Can you work these out from the model? Positions are in its coordinate system, mm. A direction names the side the tool comes from. Give positions to 0.01 mm unless a question says otherwise; leave off trailing zeros. Write each loop counter-clockwise with the first axis right and the second up, starting at its lowest first coordinate (ties: lowest second). Pieces come first, ordered by that corner, then holes.
from build123d import *

# Parameters (mm, degrees)
SKETCH1_W           = 50
SKETCH1_H           = 25
BOSS_EXTRUDE2_DEPTH = 3
SKETCH3_R           = 8.25
CUT_EXTRUDE2_DEPTH  = 29.111385594
SKETCH6_W           = 50
SKETCH6_H           = 25
SKETCH6_W_2         = 46
SKETCH6_H_2         = 21
BOSS_EXTRUDE3_DEPTH = 6
SKETCH7_W           = 50
SKETCH7_H           = 2
BOSS_EXTRUDE4_DEPTH = 12
SKETCH9_R           = 1.5
CUT_EXTRUDE3_DEPTH  = 40.937451095


with BuildPart() as part:
    # Sketch1 → Boss-Extrude2 (new body)
    with BuildSketch(Plane(origin=(0, 0, 0), x_dir=(1, 0, 0), z_dir=(0, 1, 0))):
        Rectangle(SKETCH1_W, SKETCH1_H)
    extrude(amount=BOSS_EXTRUDE2_DEPTH)

    # Sketch3 → Cut-Extrude2 (cut, through all)
    with BuildSketch(Plane(origin=(0, 3, 0), x_dir=(1, 0, 0), z_dir=(0, 1, 0))):
        with Locations(Location((13.25, 0, 0), (0, 0, 270))):
            Circle(SKETCH3_R)
        with Locations(Location((-13.25, 0, 0), (0, 0, 270))):
            Circle(SKETCH3_R)
    extrude(amount=-CUT_EXTRUDE2_DEPTH, mode=Mode.SUBTRACT)

    # Sketch6 → Boss-Extrude3 (add)
    with BuildSketch(Plane(origin=(0, 3, 0), x_dir=(1, 0, 0), z_dir=(0, 1, 0))):
        Rectangle(SKETCH6_W, SKETCH6_H)
        Rectangle(SKETCH6_W_2, SKETCH6_H_2, mode=Mode.SUBTRACT)
    extrude(amount=BOSS_EXTRUDE3_DEPTH)

    # Sketch7 → Boss-Extrude4 (add)
    with BuildSketch(Plane(origin=(0, 9, 0), x_dir=(1, 0, 0), z_dir=(0, 1, 0))):
        with Locations((0, -11.5)):
            Rectangle(SKETCH7_W, SKETCH7_H)
    extrude(amount=BOSS_EXTRUDE4_DEPTH)

    # Sketch9 → Cut-Extrude3 (cut, through all)
    with BuildSketch(Plane(origin=(0, 0, 10.5), x_dir=(-1, 0, 0), z_dir=(0, 0, -1))):
        with Locations((-15, 15.02673795)):
            Circle(SKETCH9_R)
        with Locations((15, 15.02673795)):
            Circle(SKETCH9_R)
    extrude(amount=-CUT_EXTRUDE3_DEPTH, mode=Mode.SUBTRACT)


solid = part.part
(1) Imagine slicing it at A-A, the plane z = 0. Write out the boundary of the cut face in (x, y), plus the area to 3 significant figures.
Returned:
outline: (-25, 0) - (-21.5, 0) - (-21.5, 3) - (-23, 3) - (-23, 9) - (-25, 9) - close; (-5, 0) - (5, 0) - (5, 3) - (-5, 3) - close; (21.5, 0) - (25, 0) - (25, 9) - (23, 9) - (23, 3) - (21.5, 3) - close
area: 75.0 mm2
(2) Will these pins go through, and if not, where does the flat tip stop? P1, Ø1.8, axis at x = 15, y = 15.03, coming from the +Z side; P2, Ø7, axis at x = -1, z = 2, coming from the +Y side.
Returned:
P1: passes through
P2: stops at y = 3
(3) Imagine slicing it at D-D, the plane x = 22.5. Write out the boundary of the cut face in (y, z), plus the area to 3 significant figures.
Returned:
outline: (0, -12.5) - (9, -12.5) - (9, -10.5) - (3, -10.5) - (3, 10.5) - (21, 10.5) - (21, 12.5) - (0, 12.5) - close
area: 123 mm2
(4) For faces 5 (the face through (5.2, 1.5, -1.8)), 6 (the face through (-2, 9, -11)), 7 (the face through (0, 3, 0)), which set-ups out of +Z, -Z, +X, -X, +Y, -Y let a thin tool reach every point of the face, with its end or its side?
Returned:
face 5: +Y, -Y
face 6: -Z, +X, -X, +Y
face 7: +Y
(5) If we mould it in two halves opening along X, with no side actions, what happens to faces 1 (the face through (23, 6, 0)), 2 (the face through (0, 6, -10.5)), 3 (the face through (0, 0, 0)), 4 (the face through (25, 6, 0))? For each: +X half, -X half, draft (parallel to the pull), parting line (faces both ways), or undercut.
Returned:
face 1: undercut
face 2: undercut
face 3: draft
face 4: +X half
(6) If I drill on L1, parallel to X at y = 1.5, z = 0; L2, parallel to Y at x = 15, z = 11.7; L3, parallel to X at y = 2.25, z = -4, over which ranges is the centre line in solid material (lowest first)?
Returned:
L1: x = -25 to -21.5, -5 to 5, 21.5 to 25
L2: y = 0 to 13.53, 16.53 to 21
L3: x = -25 to -20.47, -6.03 to 6.03, 20.47 to 25
(7) Imagine slicing it at C-C, the plane y = 7.5. Write out the boundary of the cut face in (x, z), plus the area to 3 significant figures.
Returned:
outline: (-25, -12.5) - (25, -12.5) - (25, 12.5) - (-25, 12.5) - close; hole (-23, -10.5) - (23, -10.5) - (23, 10.5) - (-23, 10.5) - close
area: 284 mm2
(8) Imagine slicing it at B-B, the plane x = -11. Write out the boundary of the cut face in (y, z), plus the area to 3 significant figures.
Returned:
outline: (0, -12.5) - (9, -12.5) - (9, -10.5) - (3, -10.5) - (3, -7.94) - (0, -7.94) - close; (0, 7.94) - (3, 7.94) - (3, 10.5) - (21, 10.5) - (21, 12.5) - (0, 12.5) - close
area: 75.4 mm2
